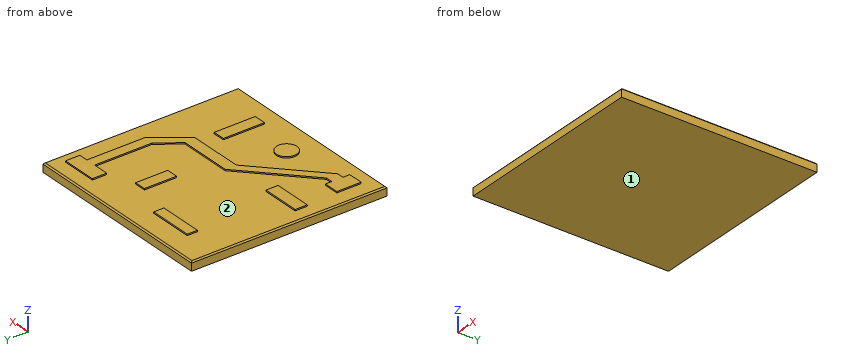
```python
from build123d import *

# Parameters (mm, degrees)
F0_W     = 38.1
F0_H     = 38.1
F1_DEPTH = 1.7272
F2_SIZE  = 0.254
F3_W     = 8.605414
F3_H     = 1.998895
F3_W_2   = 2.356245
F3_H_2   = 7.990742
F3_W_3   = 7.478513
F3_H_3   = 2.356244
F3_W_4   = 2.253799
F3_H_4   = 6.24917
F3_R     = 1.989131
F4_DEPTH = 0.254


with BuildPart() as f1:
    # F0 (on Top) → F1 (new body)
    with BuildSketch(Plane.XY):
        Rectangle(F0_W, F0_H)
    extrude(amount=F1_DEPTH)

    # F2
    f2_edges = [f1.edges().sort_by_distance(p)[0] for p in [
        (0, -19.05, 1.7272),
        (-19.05, 0, 1.7272),
        (0, 19.05, 1.7272),
        (19.05, 0, 1.7272),
    ]]
    chamfer(f2_edges, length=F2_SIZE)

    # F3 (on face) → F4 (join)
    with BuildSketch(Plane.XY.offset(1.7272)):
        Polygon((-13.00328, -11.657394), (-15.904149, -11.657394), (-15.904149, -16.395478), (-13.00328, -16.395478), (-13.00328, -15.04174), (-13.00328, -14.026436), (-13.00328, -12.888039), align=None)
        Polygon((-11.649542, -12.888039), (-13.00328, -12.888039), (-13.00328, -14.026436), (-11.649542, -14.026436), (0, -3.118129), (10.672469, -3.118129), (14.540292, 2.151779), (14.540292, 11.33786), (14.540292, 13.368469), (13.28325, 13.368469), (13.28325, 11.33786), (13.28325, 2.151779), (10.250947, -1.979733), (0, -1.979733), align=None)
        Polygon((-11.649542, -14.026436), (-13.00328, -14.026436), (-13.00328, -15.04174), (-11.649542, -15.04174), (0, -4.133433), (10.672469, -4.133433), (15.274137, 2.136338), (15.274137, 11.51581), (15.274137, 13.368469), (14.540292, 13.368469), (14.540292, 11.33786), (14.540292, 2.151779), (10.672469, -3.118129), (0, -3.118129), align=None)
        Polygon((12.026207, 13.368469), (13.28325, 13.368469), (14.540292, 13.368469), (15.274137, 13.368469), (17.054377, 13.368469), (17.054377, 16.17264), (10.188991, 16.17264), (10.188991, 13.368469), align=None)
        with Locations((-7.976379, 13.745683)):
            Rectangle(F3_W, F3_H)
        with Locations((8.875891, -11.480894)):
            Rectangle(F3_W_2, F3_H_2)
        with Locations((-12.637645, -4.360938)):
            Rectangle(F3_W_3, F3_H_3)
        with Locations((4.009735, 8.444738)):
            Rectangle(F3_W_4, F3_H_4)
        with Locations((-1.112536, -13.120022)):
            Circle(F3_R)
    extrude(amount=F4_DEPTH)


solid = f1.part
```
Verification items for the finished model (mm, model axes). Face numbers are marked on the shaded views. Coordinates: 2 decimals unless noted, no trailing zeros. Loops run counter-clockwise (first coordinate to the right, second up) from the corner with the lowest first, then second, coordinate; pieces in that order, holes last. Notation, with made-up numbers: (79, 30) - (136, 30) arc R18 ccw to (136, 59) - close; hole circle Ø2 at (73.25, -11). An arc over 180 degrees is marked (long way). Return JSON: item names as keys, results as strings.
1. Section check B-B, the plane y = 9.5. Record the boundary of the cut face in (x, z).
Established:
{"outline": "(-19.05, 0) - (19.05, 0) - (19.05, 1.47) - (18.8, 1.73) - (15.27, 1.73) - (15.27, 1.98) - (13.28, 1.98) - (13.28, 1.73) - (5.14, 1.73) - (5.14, 1.98) - (2.88, 1.98) - (2.88, 1.73) - (-18.8, 1.73) - (-19.05, 1.47) - close"}
2. Mould release check, pull along X, two halves, no side actions. Record for the marked faces 1 and 2: +X half, -X half, draft (parallel to the pull), parting line (faces both ways), or undercut.
Established:
{"face 1": "draft", "face 2": "undercut"}
3. Section check C-C, the plane x = -9.5. Record the boundary of the cut face in (y, z), then the cut area to 3 significant figures.
Established:
{"outline": "(-19.05, 0) - (19.05, 0) - (19.05, 1.47) - (18.8, 1.73) - (14.75, 1.73) - (14.75, 1.98) - (12.75, 1.98) - (12.75, 1.73) - (-3.18, 1.73) - (-3.18, 1.98) - (-5.54, 1.98) - (-5.54, 1.73) - (-10.88, 1.73) - (-10.88, 1.98) - (-13.03, 1.98) - (-13.03, 1.73) - (-18.8, 1.73) - (-19.05, 1.47) - close", "area": "67.4 mm2"}
4. Thickness scan on L1, parallel to Z at x = -12, y = 6; L2, parallel to X at y = 8.5, z = 1.6; L3, parallel to X at y = -4.5, z = 1.5. Record the ranges inside material, lowest first.
Established:
{"L1": "z = 0 to 1.73", "L2": "x = -18.92 to 18.92", "L3": "x = -19.02 to 19.02"}
5. Section check D-D, the plane y = -14. Record the boundary of the cut face in (x, z), then the cut area to 3 significant figures.
Established:
{"outline": "(-19.05, 0) - (19.05, 0) - (19.05, 1.47) - (18.8, 1.73) - (10.05, 1.73) - (10.05, 1.98) - (7.7, 1.98) - (7.7, 1.73) - (0.67, 1.73) - (0.67, 1.98) - (-2.9, 1.98) - (-2.9, 1.73) - (-10.54, 1.73) - (-10.54, 1.98) - (-15.9, 1.98) - (-15.9, 1.73) - (-18.8, 1.73) - (-19.05, 1.47) - close", "area": "68.6 mm2"}
6. Section check A-A, the plane x = -15. Record the boundary of the cut face in (y, z).
Established:
{"outline": "(-19.05, 0) - (19.05, 0) - (19.05, 1.47) - (18.8, 1.73) - (-3.18, 1.73) - (-3.18, 1.98) - (-5.54, 1.98) - (-5.54, 1.73) - (-11.66, 1.73) - (-11.66, 1.98) - (-16.4, 1.98) - (-16.4, 1.73) - (-18.8, 1.73) - (-19.05, 1.47) - close"}
7. Go/stop test with a flat-tipped pin: pin 1 (2 mm diameter, centred on x = 7, y = -0.5, fed in from +Z). Record where the tip stops, or that it passes through.
Established:
{"pin 1": "stops at z = 1.73"}
